Could you check a few things on this model? Use its own coordinates, in mm. Coordinates: 2 decimals unless noted, no trailing zeros. Order: outer loops, then holes, each group sorted by start corner. A loop starts at its lowest first (then second) coordinate and runs counter-clockwise, first axis right, second up. Notation, with made-up numbers: (-21.75, -18.75) -> (-17.75, -18.75) arc R34 ccw to (-17.75, 19.25) -> close; hole circle Ø3 at (66.5, -20). An arc over 180 degrees is marked (long way). Put each result on its own line as item: value. Start each with the question number.
Q1. If we section it at C-C (y = -132): Please give me the cut outline in (x, z), and give its area (3 significant figures).
Q2. If we section it at D-D (x = 124): Please give me the cut outline in (y, z).
Q3. If we section it at A-A (x = 95): Please give me the cut outline in (y, z), and give its area (3 significant figures).
Q4. Please list where these lines run through material, in increasing order: line 1 along Y through (x, z) = (92.5, 5); line 2 along Y through (x, z) = (44, 2.75); line 3 along X through (y, z) = (-93, 2.5).
Q5. Will these pins go through, and if not, where does the flat tip stop? pin 1 (6.5 mm diameter, centred on x = 170.734, y = -21, fed in from +Z); pin 2 (9.5 mm diameter, centred on x = 95.734, y = -21, fed in from +Z); pin 3 (2 mm diameter, centred on x = 96, z = 7, fed in from -Y); pin 4 (2 mm diameter, centred on x = 115.5, z = 4, fed in from -Y).
Q6. We'd pull the mould along X, two halves only. Please class faces 1 (the face through (183.234, -4, 6)), 2 (the face through (70, -83, 0)), 3 (the face through (169.856, -17.046, 6.286)): +X half, -X half, draft (parallel to the pull), parting line (faces both ways), or undercut.
Q7. If we section it at B-B (z = 2.75): Please give me the cut outline in (x, y), and give its area (3 significant figures).
Autodesk Inventor part; units mm, degrees
ref_plane "YZ Plane" through (0, 0, 0) normal (1, 0, 0) x (0, 1, 0)
ref_plane "XZ Plane" through (0, 0, 0) normal (0, 1, 0) x (-1, 0, 0)
ref_plane "XY Plane" through (0, 0, 0) normal (0, 0, 1) x (1, 0, 0)
ref_plane "Work Plane1" through (0, 0, 0) normal (0, 0, 1) x (1, 0, 0)
sketch "Sketch1" plane through (0, 0, 0) normal (0, 0, 1) x (1, 0, 0)
  circle A0 centre (95.734, -21) radius 4.05
  circle A1 centre (170.734, -21) radius 4.05
  line L0 (78.234, -5) -> (78.234, 0)
  arc A2 (83.234, -10) -> (78.234, -5) centre (78.234, -10) ccw
  line L1 (83.234, -10) -> (83.234, -21)
  arc A3 (83.234, -21) -> (108.234, -21) centre (95.734, -21) ccw
  line L2 (108.234, -21) -> (108.234, -10)
  arc A4 (113.234, -5) -> (108.234, -10) centre (113.234, -10) ccw
  line L3 (113.234, -5) -> (153.234, -5)
  arc A5 (158.234, -10) -> (153.234, -5) centre (153.234, -10) ccw
  line L4 (158.234, -10) -> (158.234, -21)
  arc A6 (158.234, -21) -> (183.234, -21) centre (170.734, -21) ccw
  line L5 (183.234, -21) -> (183.234, -10)
  arc A7 (188.234, -5) -> (183.234, -10) centre (188.234, -10) ccw
  line L6 (188.234, 0) -> (188.234, -5)
  line L7 (78.234, 0) -> (188.234, 0)
  line L8 (437.5, 12.7) -> (437.5, 0)
  line L9 (0, 12.7) -> (437.5, 12.7)
  line L10 (0, 0) -> (0, 12.7)
  line L11 (437.5, 0) -> (0, 0)
  line L12 (0, 12.7) -> (0, -237.3)
  line L13 (0, -237.3) -> (25, -237.3)
  line L14 (25, -237.3) -> (180.7539, -28.4734)
  line L15 (183.234, -10) -> (183.234, 12.7)
  line L16 (183.234, 12.7) -> (0, 12.7)
  dimension "d0" = 25
  dimension "d2" = 250
extrude "Extrusion1" add sketch "Sketch1" along normal blind 12.7508 contours A2 L1 A3 L2 A4 L3 A5 L4 A6 L14 L13 L12 L11 L0 | L0 L7 L15 L5 A6 L4 A5 L3 A4 L2 A3 L1 A2 | L11 L10 L9 L15 L7
properties part number "support"
The answers:
1. outline: (0, 0) -> (103.54, 0) -> (103.54, 12.75) -> (0, 12.75) -> close
1. area: 1,320 mm^2
2. outline: (-104.57, 0) -> (12.7, 0) -> (12.7, 12.75) -> (-104.57, 12.75) -> close
3. outline: (-143.45, 0) -> (-24.98, 0) -> (-24.98, 12.75) -> (-143.45, 12.75) -> close; (-17.02, 0) -> (12.7, 0) -> (12.7, 12.75) -> (-17.02, 12.75) -> close
3. area: 1,890 mm^2
4. line 1: -146.8 to -23.44, -18.56 to 12.7
4. line 2: -211.83 to 12.7
4. line 3: 0 to 132.63
5. pin 1: through
5. pin 2: z = 12.75
5. pin 3: y = -143.45
5. pin 4: y = -117.3
6. face 1: +X half
6. face 2: draft
6. face 3: undercut
7. outline: (0, -237.3) -> (25, -237.3) -> (180.75, -28.47) arc R12.5 ccw to (183.23, -21) -> (183.23, 12.7) -> (0, 12.7) -> close; hole circle Ø8.1 at (95.73, -21); hole circle Ø8.1 at (170.73, -21)
7. area: 28,900 mm^2
